Part model, mm, in its own coordinate system. A direction names the side the tool comes from. Round coordinates to 2 decimals unless told otherwise and drop trailing zeros. Loops run counter-clockwise (first coordinate to the right, second up) from the corner with the lowest first, then second, coordinate; pieces in that order, holes last. Notation, with made-up numbers: (39, 58.25) -> (44, 58.25) arc R13 ccw to (44, 64.25) -> close; hole circle Ø1 at (78, 16). An arc over 180 degrees is marked (long way). Use a Markdown table: item, result. Add a question column.
Item 1: Which spindle directions (+Z, -Z, +X, -X, +Y, -Y) get a long thin tool onto all of the face, cutting with end or side? Do faces 4 (the face through (16.942, 2, -6)), 5 (the face through (15.428, 1.61, -43.806)). Say none if no direction does.
Item 2: Probe line 1 (X direction, y = 0.7, z = -3); line 2 (Z direction, x = -14.5, y = 0.4) (3 decimals); line 3 (X direction, y = 3, z = -30). List the from-to ranges inside material, lowest first. Write a range as [from, to].
Item 3: Cut at A-A, the plane x = 0. State how many separate pieces and enclosed holes the cut face has, plus the area to 3 significant figures.
Item 4: Cut at C-C, the plane z = -23. List the corners of the cut face in (x, y) (3 decimals), plus the area to 3 significant figures.
Item 5: Cut at D-D, the plane x = -16. List the corners of the cut face in (y, z) (3 decimals).
Item 6: Cut at B-B, the plane z = -5. List the corners of the cut face in (x, y) (3 decimals).
Item 7: Two-plate mould, pull along Z, no slides. Class faces 1 (the face through (0, 2, -11.588)), 2 (the face through (0, 2, 6.35)), 3 (the face through (19.05, 2, -14)): pulls with the +Z half, pulls with the -Z half, needs draft (parallel to the pull), parting line crosses it, or undercut.
Autodesk Inventor part; units mm, degrees
ref_plane "XZ Plane" through (0, 0, 0) normal (0, 1, 0) x (-1, 0, 0)
ref_plane "XY Plane" through (0, 0, 0) normal (0, 0, 1) x (1, 0, 0)
sketch "Sketch1" plane through (0, 0, 0) normal (0, 1, 0) x (-1, 0, 0)
  line L0 (-9.2075, -1.5875) -> (9.2075, -1.5875)
  line L1 (9.2075, -1.5875) -> (9.2075, 1.5875)
  line L2 (9.2075, 1.5875) -> (-9.2075, 1.5875)
  line L3 (-9.2075, 1.5875) -> (-9.2075, -1.5875)
  line L4 (-9.2075, -1.5875) -> (9.2075, 1.5875) construction
  line L5 (9.2075, -1.5875) -> (-9.2075, 1.5875) construction
  line L6 (-9.2075, -6.5875) -> (9.2075, -6.5875)
  line L7 (9.2075, -6.5875) -> (9.2075, -3.4125)
  line L8 (9.2075, -3.4125) -> (-9.2075, -3.4125)
  line L9 (-9.2075, -3.4125) -> (-9.2075, -6.5875)
  line L10 (-9.2075, -6.5875) -> (9.2075, -3.4125) construction
  line L11 (9.2075, -6.5875) -> (-9.2075, -3.4125) construction
  line L12 (-9.2075, -11.5875) -> (9.2075, -11.5875)
  line L13 (9.2075, -11.5875) -> (9.2075, -8.4125)
  line L14 (9.2075, -8.4125) -> (-9.2075, -8.4125)
  line L15 (-9.2075, -8.4125) -> (-9.2075, -11.5875)
  line L16 (-9.2075, -11.5875) -> (9.2075, -8.4125) construction
  line L17 (9.2075, -11.5875) -> (-9.2075, -8.4125) construction
  line L18 (19.05, 6.35) -> (-19.05, 6.35)
  line L19 (-19.05, 6.35) -> (-19.05, -47.625)
  line L20 (-19.05, -47.625) -> (19.05, -47.625)
  line L21 (19.05, -47.625) -> (19.05, 6.35)
  circle A0 centre (0, -30.1625) radius 16.6687
  circle A1 centre (9.2075, 0) radius 1.5875
  circle A2 centre (9.2075, -5) radius 1.5875
  circle A3 centre (9.2075, -10) radius 1.5875
  circle A4 centre (-9.2075, -10) radius 1.5875
  circle A5 centre (-9.2075, -5) radius 1.5875
  circle A6 centre (-9.2075, 0) radius 1.5875
  line L22 (14.9225, 0) -> (14.9225, -12.7) construction
  line L23 (12.9032, 0) -> (12.9032, -12.7)
  line L24 (16.9418, -12.7) -> (16.9418, 0)
  arc A7 (16.9418, 0) -> (12.9032, 0) centre (14.9225, 0) ccw
  arc A8 (12.9032, -12.7) -> (16.9418, -12.7) centre (14.9225, -12.7) ccw
  line L25 (-14.9225, 0) -> (-14.9225, -12.7) construction
  line L26 (-16.9418, 0) -> (-16.9418, -12.7)
  line L27 (-12.9032, -12.7) -> (-12.9032, 0)
  arc A9 (-12.9032, 0) -> (-16.9418, 0) centre (-14.9225, 0) ccw
  arc A10 (-16.9418, -12.7) -> (-12.9032, -12.7) centre (-14.9225, -12.7) ccw
  line L28 (10.795, 0) -> (19.05, 0) construction
  line L29 (-10.795, 0) -> (-19.05, 0) construction
  point P0 (0, 0)
  point P1 (0, -5)
  point P2 (0, -10)
  point P3 (0, 6.35)
  point P4 (-9.2075, -11.5875)
  point P5 (9.2075, -8.4125)
  point P6 (-9.2075, -1.5875)
  point P7 (9.2075, 1.5875)
  point P8 (-9.2075, -6.5875)
  point P9 (9.2075, -3.4125)
  point P10 (14.9225, -6.35)
  point P11 (-14.9225, -6.35)
  point P12 (14.9225, 0)
  point P13 (-14.9225, 0)
  dimension "d0" = 18.415
  dimension "d1" = 3.175
  dimension "d6" = 5
  dimension "d7" = 5
  dimension "d8" = 38.1
  dimension "d9" = 53.975
  dimension "d10" = 6.35
  dimension "d11" = 33.3375
  dimension "d20" = 17.4625
  dimension "d21" = 4.0386
  dimension "d22" = 4.0386
  dimension "d23" = 12.7
  dimension "d26" = 12.7
extrude "Extrusion1" add sketch "Sketch1" along normal blind 3.175
sketch "Sketch2" plane through (0, 3.175, 0) normal (0, 1, 0) x (1, 0, 0)
  circle A0 centre (0, 45.085) radius 2.286
  line L0 (19.05, 47.625) -> (-19.05, 47.625)
  point P0 (0, 0)
  point P1 (0, 47.625)
  dimension "d14" = 4.572
  dimension "d15" = 2.54
extrude "Extrusion2" add sketch "Sketch2" against normal blind 3.175
fillet "Fillet1" radius 3.175 2 edges at (-1.5575, 1.5875, -46.7583) (1.5575, 1.5875, -46.7583)
fillet "Fillet2" radius 12.7 2 edges at (-19.05, 1.5875, -47.625) (19.05, 1.5875, -47.625)
equation "\"d21\" = d22"
properties part number "EL2-018" material "Aluminum 6061"
A:
| question | item | result |
|---|---|---|
| 1 | face 4 | +Y, -Y |
| 1 | face 5 | -Z, +X, +Y, -Y |
| 2 | line 1 | x = [-19.05, -16.94], [-12.9, 12.9], [16.94, 19.05] |
| 2 | line 2 | z = [-44.665, -38.384], [-21.941, -14.675], [1.975, 6.35] |
| 2 | line 3 | x = [-19.05, -16.67], [16.67, 19.05] |
| 3 | separate pieces | 5 |
| 3 | enclosed holes | 0 |
| 3 | area | 48.1 mm^2 |
| 4 | outline | (-19.05, 0) -> (-15.051, 0) -> (-15.051, 3.175) -> (-19.05, 3.175) -> close; (15.051, 0) -> (19.05, 0) -> (19.05, 3.175) -> (15.051, 3.175) -> close |
| 4 | area | 25.4 mm^2 |
| 5 | outline | (0, -43.181) -> (3.175, -43.181) -> (3.175, -34.836) -> (0, -34.836) -> close; (0, -25.489) -> (3.175, -25.489) -> (3.175, -14.408) -> (0, -14.408) -> close; (0, 1.708) -> (3.175, 1.708) -> (3.175, 6.35) -> (0, 6.35) -> close |
| 6 | outline | (-19.05, 0) -> (-16.942, 0) -> (-16.942, 3.175) -> (-19.05, 3.175) -> close; (-12.903, 0) -> (-10.795, 0) -> (-10.795, 3.175) -> (-12.903, 3.175) -> close; (10.795, 0) -> (12.903, 0) -> (12.903, 3.175) -> (10.795, 3.175) -> close; (16.942, 0) -> (19.05, 0) -> (19.05, 3.175) -> (16.942, 3.175) -> close |
| 7 | face 1 | undercut |
| 7 | face 2 | pulls with the +Z half |
| 7 | face 3 | needs draft |
